```python
from build123d import *

# Parameters (mm, degrees)
F1_DEPTH = 10
F2_T     = -2
F5_DEPTH = 4
F6_R     = 13.5
F7_DEPTH = 20
F8_R     = 4
F9_DEPTH = 20
F11_D    = 6
F12_R    = 2
F13_R    = 2


with BuildPart() as f1:
    # F0 (on Front) → F1 (new body)
    with BuildSketch(Plane.XZ):
        Polygon((0, 154), (0, 0), (275, 0), (275, 80), (201, 154), align=None)
    extrude(amount=F1_DEPTH)

    # F2
    f2_openings = [f1.faces().sort_by_distance(p)[0] for p in [
        (129.700907, 0, 73.382695),
    ]]
    offset(amount=F2_T, openings=f2_openings)

    # F4 (on face) → F5 (join)
    with BuildSketch(Plane(origin=(0, -8, 0), x_dir=(-1, 0, 0), z_dir=(0, 1, 0))):
        Polygon((-32, 87), (-32, 132), (-177, 132), (-177, 22), (-97, 22), align=None)
    extrude(amount=F5_DEPTH)

    # F6 (on face) → F7 (join)
    with BuildSketch(Plane(origin=(0, -8, 0), x_dir=(-1, 0, 0), z_dir=(0, 1, 0))):
        with Locations((-44, 44)):
            Circle(F6_R)
    extrude(amount=F7_DEPTH)

    # F8 (on face) → F9 (cut, through all)
    with BuildSketch(Plane(origin=(0, 12, 0), x_dir=(-1, 0, 0), z_dir=(0, 1, 0))):
        with Locations((-44, 44)):
            Circle(F8_R)
    extrude(amount=-F9_DEPTH, mode=Mode.SUBTRACT)

    # F11 (through all)
    with Locations(Plane.XZ.offset(10)):
        with Locations((9.5, 144.5), (109.5, 144.5), (231.2824855787, 110.2824855787), (265.5, 9.5), (137.5, 9.5), (9.5, 9.5)):
            Hole(F11_D / 2)

    # F12
    f12_edges = [f1.edges().sort_by_distance(p)[0] for p in [
        (0, -10, 77),
        (137.5, -10, 0),
        (238, -10, 117),
        (275, -10, 40),
        (275, -5, 0),
        (275, -5, 80),
        (201, -5, 154),
        (0, -5, 0),
        (100.5, -10, 154),
        (0, -5, 154),
    ]]
    fillet(f12_edges, radius=F12_R)

    # F13
    f13_edges = [f1.edges().sort_by_distance(p)[0] for p in [
        (273, -4, 2),
        (137.5, -8, 2),
        (273, -8, 40.585786),
        (236.585786, -8, 115.585786),
        (200.171573, -4, 152),
        (101.085786, -8, 152),
        (2, -4, 2),
        (2, -8, 77),
    ]]
    fillet(f13_edges, radius=F13_R)


solid = f1.part
```
Input: part model. Units: mm. Frame: model coordinates. A direction names the side the tool comes from. Give positions to 0.01 mm unless a question says otherwise; leave off trailing zeros. Write each loop counter-clockwise with the first axis right and the second up, starting at its lowest first coordinate (ties: lowest second). Pieces come first, ordered by that corner, then holes. Notation, with made-up numbers: (-29.5, 43.5) - (9.5, 43.5) arc R24 ccw to (9.5, 63.5) - close; hole circle Ø4 at (89.5, 47.25). An arc over 180 degrees is marked (long way). Write item = value, one per line. Start each with the question number.
1. Ray query, L1, parallel to Z at x = 9.5, y = -8.5; L2, parallel to Z at x = 102.5, y = -2.5; L3, parallel to X at y = -3.25, z = 73. Return the intervals inside material, ascending.
2. First-contact query: pin 1 Ø6 at (y, z) = (1, 97) entering from +X; pin 2 Ø5 at (y, z) = (-3, 94) entering from +X; pin 3 Ø12 at (x, z) = (91, 59) entering from +Y; pin 4 Ø6.5 at (x, z) = (45.5, 42.5) entering from +Y. Flat tips, straight axial feed; report the tip coordinate or a pass-through.
3. Mould query, pull axis Z, two halves, no side actions, for faces 1 (the cylindrical face through (237.065, -9.43, 117.085)), 2 (the flat face through (136, -4, 0)), 3 (the flat face through (102, -3, 152)). Classes: released by +Z, released by -Z, zero draft, split by the parting line, or undercut.
4. Access query for faces 4 (the cylindrical face through (7.89, -8.99, 147.03)), 5 (the flat face through (106, -4, 78)). Directions: +Z, -Z, +X, -X, +Y, -Y. A direction counts if a zero-diameter tool reaches every point of the face in a straight line with its end or side. Return the directions, or none.
5. Section query D-D, the plane z = 64. Output: boundary loops of the cut face in (x, y), then the cut area to 3 significant figures.
6. Section query A-A, the plane x = 9.5. Output: boundary loops of the cut face in (y, z), then the cut area to 3 significant figures.
7. Section query C-C, the plane x = 144. Output: boundary loops of the cut face in (y, z).
8. Section query B-B, the plane x = 109.5. Output: boundary loops of the cut face in (y, z).
Check sheet entries:
q1.L1 = 0.06 to 6.5, 12.5 to 141.5, 147.5 to 153.94
q1.L2 = 0 to 2, 152 to 154
q1.L3 = 0 to 2, 273 to 275
q2.pin_1 = 260.83
q2.pin_2 = 263.5
q2.pin_3 = -4
q2.pin_4 = 12
q3.face_1 = released by +Z
q3.face_2 = released by -Z
q3.face_3 = undercut
q4.face_4 = +Y, -Y
q4.face_5 = +Y
q5.outline = (0, -8) arc R2 ccw to (2, -10) - (273, -10) arc R2 ccw to (275, -8) - (275, 0) - (273, 0) - (273, -6) arc R2 cw to (271, -8) - (177, -8) - (177, -4) - (55, -4) - (55, -8) - (4, -8) arc R2 cw to (2, -6) - (2, 0) - (0, 0) - close
q5.area = 1,070 mm2
q6.outline = (-10, 2) arc R2 ccw to (-8, 0) - (0, 0) - (0, 2) - (-6, 2) arc R2 cw to (-8, 4) - (-8, 6.5) - (-10, 6.5) - close; (-10, 12.5) - (-8, 12.5) - (-8, 141.5) - (-10, 141.5) - close; (-10, 147.5) - (-8, 147.5) - (-8, 150) arc R2 cw to (-6, 152) - (0, 152) - (0, 154) - (-8, 154) arc R2 ccw to (-10, 152) - close
q6.area = 316 mm2
q7.outline = (-10, 2) arc R2 ccw to (-8, 0) - (0, 0) - (0, 2) - (-6, 2) arc R2 cw to (-8, 4) - (-8, 22) - (-4, 22) - (-4, 132) - (-8, 132) - (-8, 150) arc R2 cw to (-6, 152) - (0, 152) - (0, 154) - (-8, 154) arc R2 ccw to (-10, 152) - close
q8.outline = (-10, 2) arc R2 ccw to (-8, 0) - (0, 0) - (0, 2) - (-6, 2) arc R2 cw to (-8, 4) - (-8, 22) - (-4, 22) - (-4, 132) - (-8, 132) - (-8, 141.5) - (-10, 141.5) - close; (-10, 147.5) - (-8, 147.5) - (-8, 150) arc R2 cw to (-6, 152) - (0, 152) - (0, 154) - (-8, 154) arc R2 ccw to (-10, 152) - close
